The model under review builds one solid part; all positions refer to its coordinate system, in mm. A direction names the side the tool comes from. Coordinates: 2 decimals unless noted, no trailing zeros. Write each loop counter-clockwise with the first axis right and the second up, starting at its lowest first coordinate (ties: lowest second). Pieces come first, ordered by that corner, then holes. Notation, with made-up numbers: (49.5, -14) - (55.5, -14) arc R35 ccw to (55.5, 22) - close; hole circle Ø8 at (59.25, -22.5). An arc over 180 degrees is marked (long way). Put each result on its own line as item: value.
from build123d import *

# Parameters (mm, degrees)
BOSS_EXTRUDE1_DEPTH = 3.048
SKETCH2_W           = 4.572
SKETCH2_H           = 5.08
SKETCH2_W_2         = 5.08
SKETCH2_H_2         = 2.54
SKETCH2_W_3         = 2.54
SKETCH2_H_3         = 4.572
SKETCH2_R           = 2.54
CUT_EXTRUDE1_DEPTH  = 3.048
SKETCH3_W           = 16.002
SKETCH3_H           = 16.002
CUT_EXTRUDE2_DEPTH  = 3.048


with BuildPart() as part:
    # Sketch1 → Boss-Extrude1 (new body)
    with BuildSketch(Plane(origin=(0, 0, 0), x_dir=(1, 0, 0), z_dir=(0, 1, 0))):
        Polygon((0, 19.05), (0, 0), (19.05, 0), (19.05, 3.048), (31.75, 3.048), (31.75, 0), (47.752, 0), (47.752, 19.05), (50.8, 19.05), (50.8, 31.75), (47.752, 31.75), (47.752, 47.752), (31.75, 47.752), (31.75, 50.8), (19.05, 50.8), (19.05, 47.752), (0, 47.752), (0, 31.75), (3.048, 31.75), (3.048, 19.05), align=None)
    extrude(amount=BOSS_EXTRUDE1_DEPTH)

    # Sketch2 → Cut-Extrude1 (cut)
    with BuildSketch(Plane(origin=(0, 3.048, 0), x_dir=(1, 0, 0), z_dir=(0, 1, 0))):
        with Locations((5.334, 25.4)):
            Rectangle(SKETCH2_W, SKETCH2_H)
        with Locations((10.16, 25.4)):
            Rectangle(SKETCH2_W_2, SKETCH2_H)
        with Locations((10.16, 29.21)):
            Rectangle(SKETCH2_W_2, SKETCH2_H_2)
        with Locations((13.97, 25.4)):
            Rectangle(SKETCH2_W_3, SKETCH2_H)
        with Locations((10.16, 21.59)):
            Rectangle(SKETCH2_W_2, SKETCH2_H_2)
        with Locations((25.4, 13.97)):
            Rectangle(SKETCH2_W_2, SKETCH2_H_2)
        with Locations((25.4, 10.16)):
            Rectangle(SKETCH2_W_2, SKETCH2_H)
        with Locations((29.21, 10.16)):
            Rectangle(SKETCH2_W_3, SKETCH2_H)
        with Locations((21.59, 10.16)):
            Rectangle(SKETCH2_W_3, SKETCH2_H)
        with Locations((25.4, 5.334)):
            Rectangle(SKETCH2_W_2, SKETCH2_H_3)
        with Locations(Location((46.99, 25.4, 0), (0, 0, 270))):
            Circle(SKETCH2_R)
        with Locations(Location((25.4, 46.99, 0), (0, 0, 270))):
            Circle(SKETCH2_R)
    extrude(amount=-CUT_EXTRUDE1_DEPTH, mode=Mode.SUBTRACT)

    # Sketch3 → Cut-Extrude2 (cut)
    with BuildSketch(Plane(origin=(0, 3.048, 0), x_dir=(1, 0, 0), z_dir=(0, 1, 0))):
        with Locations((39.751, 39.751)):
            Rectangle(SKETCH3_W, SKETCH3_H)
    extrude(amount=-CUT_EXTRUDE2_DEPTH, mode=Mode.SUBTRACT)


solid = part.part
1. For pin 1 Ø1.5 at (y, z) = (1.5, -1.5) entering from -X; pin 2 Ø1 at (x, y) = (18, 0.5) entering from -Z; pin 3 Ø1.5 at (y, z) = (2, -26) entering from -X; pin 4 Ø1.5 at (y, z) = (1.5, -15) entering from +X, all flat-tipped, find the tip position at first contact; note any pin that passes through.
Determined:
pin 1: stops at x = 0
pin 2: stops at z = -47.75
pin 3: stops at x = 15.24
pin 4: stops at x = 47.75
2. Consider section C-C on y = 1.85. Give the number of separate pieces and of enclosed holes in the cut face, plus the area to 3 significant figures.
Determined:
separate pieces: 1
enclosed holes: 2
area: 1,810 mm^2
3. Consider section B-B on z = -46.99. State the section outline as (x, y) points.
Determined:
outline: (0, 0) - (22.86, 0) - (22.86, 3.05) - (0, 3.05) - close; (27.94, 0) - (31.75, 0) - (31.75, 3.05) - (27.94, 3.05) - close
4. Consider section D-D on x = 16. State the section outline as (y, z) points.
Determined:
outline: (0, -47.75) - (3.05, -47.75) - (3.05, 0) - (0, 0) - close
5. Consider section A-A on x = 46.99. State the section outline as (y, z) points, plus the area to 3 significant figures.
Determined:
outline: (0, -31.75) - (3.05, -31.75) - (3.05, -27.94) - (0, -27.94) - close; (0, -22.86) - (3.05, -22.86) - (3.05, 0) - (0, 0) - close
area: 81.3 mm^2
6. Machinability: for faces 1 (the flat face through (30.48, 2, -10)), 2 (the flat face through (30, 2, -3.048)), 3 (the flat face through (49, 2, -19.05)), 4 (the flat face through (50.8, 2, -25)), 5 (the flat face through (14, 2, -22.86)), which of the approach directions +Z, -Z, +X, -X, +Y, -Y give a long, thin tool a straight path to every point of the face, cutting with its end or side? Answer none if there is none.
Determined:
face 1: +Y, -Y
face 2: +Z, +Y, -Y
face 3: +Z, +X, +Y, -Y
face 4: +Z, -Z, +X, +Y, -Y
face 5: -X, +Y, -Y
7. To check wall thickness, follow probe 1 along Z at (x, y) = (7.5, 0.5); probe 2 along X at (y, z) = (2.85, -12); probe 3 along X at (y, z) = (1.5, -25.4). State the ranges of each line that lie inside material, in increasing order.
Determined:
probe 1: z = -47.75 to -27.94, -22.86 to 0
probe 2: x = 0 to 20.32, 30.48 to 47.75
probe 3: x = 15.24 to 44.45, 49.53 to 50.8
8. The part is to be moulded in two halves that separate along Z. For faces 6 (the flat face through (20.32, 2, -10)), 7 (the flat face through (25, 2, -15.24)), 8 (the flat face through (41, 2, -31.75)), 9 (the flat face through (29, 2, -12.7)), say which applies: +Z half, -Z half, draft (parallel to the pull), parting line (faces both ways), or undercut.
Determined:
face 6: undercut
face 7: +Z half
face 8: -Z half
face 9: undercut
